```python
from build123d import *

# Parameters (mm, degrees)
CROQUIS3_W              = 0.5
CROQUIS3_H              = 0.25
SALIENTE_EXTRUIR1_DEPTH = 10


with BuildPart() as part:
    # Croquis1 → Revolución1 (revolve)
    with BuildSketch(Plane.XY, mode=Mode.PRIVATE) as revoluci_n1_sk:
        with BuildLine():
            Line((0, 0), (-2.75, 0))
            Line((-2.75, 0), (-2.75, 1))
            Line((-2.75, 1), (-2.28, 1))
            Line((-2.28, 1), (-2.28, 6.32))
            ThreePointArc((-2.28, 6.32), (-1.612203461, 7.932203461), (0, 8.6))
            Line((0, 8.6), (0, 0))
        make_face()
    revolve(revoluci_n1_sk.sketch.rotate(Axis((0, -55.273367698, 0), (0, 1, 0)), 270), axis=Axis((0, -55.273367698, 0), (0, 1, 0)))

    # Croquis3 → Saliente-Extruir1 (add)
    with BuildSketch(Plane.XZ):
        with Locations((-0.5, 0)):
            Rectangle(CROQUIS3_W, CROQUIS3_H)
        with Locations((-1.77, 0)):
            Rectangle(CROQUIS3_W, CROQUIS3_H)
        with Locations((1.77, 0)):
            Rectangle(CROQUIS3_W, CROQUIS3_H)
        with Locations((0.5, 0)):
            Rectangle(CROQUIS3_W, CROQUIS3_H)
    extrude(amount=SALIENTE_EXTRUIR1_DEPTH)


solid = part.part
```
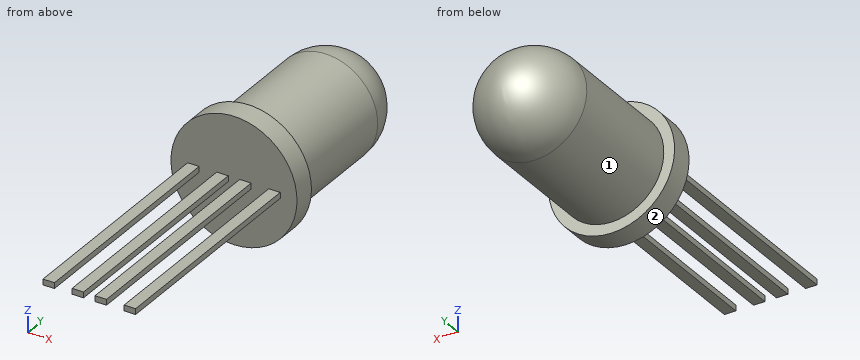
Part model, mm, in its own coordinate system. Face numbers are marked on the shaded views. A direction names the side the tool comes from. Coordinates: 2 decimals unless noted, no trailing zeros. Order: outer loops, then holes, each group sorted by start corner. A loop starts at its lowest first (then second) coordinate and runs counter-clockwise, first axis right, second up. Notation, with made-up numbers: (74, -24) - (95, -24) arc R29 ccw to (95, 12) - close; hole circle Ø9 at (88.25, 55). An arc over 180 degrees is marked (long way). Return JSON: item names as keys, results as strings. Group by question number.
Item 1: Cut at D-D (y = 5.5). List the corners of the cut face in (x, z), plus the area to 3 significant figures.
Item 2: Drill centre lines: probe 1 along X at (y, z) = (5.5, -0.1); probe 2 along Z at (x, y) = (0.45, -4.5) (3 decimals); probe 3 along Y at (x, z) = (-1.7, -1.65). Where is each one in solid material? Low to high. Write a range as from..to.
Item 3: Cut at A-A (y = -7.5). List the corners of the cut face in (x, z) (3 decimals).
Item 4: Cut at B-B (x = 0). List the corners of the cut face in (y, z), plus the area to 3 significant figures.
Item 5: Which spindle directions (+Z, -Z, +X, -X, +Y, -Y) get a long thin tool onto all of the face, cutting with end or side? Do the marked faces 1 and 2. Say none if no direction does.
Item 6: Cut at C-C (z = 1.6). List the corners of the cut face in (x, y), plus the area to 3 significant figures.
Item 7: Pin check, flat tips, straight feed: pin 1 (2 mm diameter, centred on y = -5, z = -1, fed in from -X); pin 2 (1 mm diameter, centred on x = -0.5, y = 4, fed in from +Z); pin 3 (0.6 mm diameter, centred on x = -0.5, y = -3.5, fed in from +Z) (3 decimals). Stop position of each tip, or through.
Check values:
{
 "1": {"outline": "circle Ø4.56 at (0, 0)", "area": "16.3 mm2"},
 "2": {"probe 1": "x = -2.28..2.28", "probe 2": "z = -0.125..0.125", "probe 3": "y = 0..1"},
 "3": {"outline": "(-2.02, -0.125) - (-1.52, -0.125) - (-1.52, 0.125) - (-2.02, 0.125) - close; (-0.75, -0.125) - (-0.25, -0.125) - (-0.25, 0.125) - (-0.75, 0.125) - close; (0.25, -0.125) - (0.75, -0.125) - (0.75, 0.125) - (0.25, 0.125) - close; (1.52, -0.125) - (2.02, -0.125) - (2.02, 0.125) - (1.52, 0.125) - close"},
 "4": {"outline": "(0, -2.75) - (1, -2.75) - (1, -2.28) - (6.32, -2.28) arc R2.28 ccw to (6.32, 2.28) - (1, 2.28) - (1, 2.75) - (0, 2.75) - close", "area": "37.9 mm2"},
 "5": {"face 1": "+Y", "face 2": "+Y, -Y"},
 "6": {"outline": "(-2.24, 0) - (2.24, 0) - (2.24, 1) - (1.62, 1) - (1.62, 6.32) arc R1.62 ccw to (-1.62, 6.32) - (-1.62, 1) - (-2.24, 1) - close", "area": "25.9 mm2"},
 "7": {"pin 1": "stops at x = -2.02", "pin 2": "stops at z = 2.28", "pin 3": "stops at z = 0.125"}
}
